Work out the finished part from the listing and answer in its coordinate system (mm). A direction names the side the tool comes from. Coordinates: 2 decimals unless noted, no trailing zeros. Order: outer loops, then holes, each group sorted by start corner. A loop starts at its lowest first (then second) coordinate and runs counter-clockwise, first axis right, second up. Notation, with made-up numbers: M 68.5,77.5 L 119.5,77.5 A12 ccw 119.5,83.5 Z; hole C 5,-29 d3. An arc over 180 degrees is marked long. Answer in a Markdown table with one row per item. Add a question column.
Item 1: Which of the six approach directions +Z, -Z, +X, -X, +Y, -Y give full straight-line access (tool end or side, diameter ignored) to faces 1 (the face through (9.5, 12, -23)), 2 (the face through (32, 15.25, -23)), 3 (the face through (0, 5.5, -23)), 4 (the face through (18, 15.75, -23))?
Item 2: Consider line 1 (X direction, y = 0.25, z = -9); line 2 (Z direction, x = 22, y = 18.25); line 3 (X direction, y = 16.65, z = -8). Determine where each line is inside the solid, lowest interval first. Write a range as from..to.
Item 3: The part is cut by section C-C (x = -4). Write down the section's boundary in (y, z), then the cut area to 3 significant figures.
Item 4: Flat-ended cylindrical pins translate along their axes: pin 1 Ø3.5 at (x, z) = (8, -19.5) entering from -Y; pin 2 Ø1.2 at (y, z) = (14.5, -13.5) entering from +X; pin 3 Ø1 at (x, z) = (13.5, -29) entering from -Y. Find the tip coordinate at first contact, or state that the pin passes through.
Item 5: The part is cut by section A-A (y = 0). Write down the section's boundary in (x, z).
Item 6: The mould has two halves that part along X. Classify faces 5 (the face through (12.5, 9, -23)), 6 (the face through (30, 13.75, -23)), 7 (the face through (9.5, -1, -23)): released by +X, released by -X, zero draft, split by the parting line, or undercut.
Item 7: The part is cut by section B-B (z = -8). State how many separate pieces and enclosed holes the cut face has, then the cut area to 3 significant figures.
Autodesk Inventor part; units mm, degrees
ref_plane "YZ Plane" through (0, 0, 0) normal (1, 0, 0) x (0, 1, 0)
ref_plane "XZ Plane" through (0, 0, 0) normal (0, 1, 0) x (-1, 0, 0)
ref_plane "XY Plane" through (0, 0, 0) normal (0, 0, 1) x (1, 0, 0)
sketch "Boceto1" plane through (0, 0, 0) normal (0, 0, 1) x (1, 0, 0)
  arc A0 (4.8153, 5.75) -> (4.8153, -5.75) centre (0, 0) ccw
  line L0 (0, 12.1119) -> (0, -11.4197) construction
  line L1 (-11.1817, 0) -> (12.1806, 0) construction
  line L2 (4.9434, 0.75) -> (5.5, 0.75)
  line L3 (4.9434, -0.75) -> (5.5, -0.75)
  line L4 (5.5, -0.75) -> (5.5, 0.75)
  line L5 (-0.75, 4.9434) -> (-0.75, 5.5)
  line L6 (0.75, 5.5) -> (-0.75, 5.5)
  line L7 (0.75, 4.9434) -> (0.75, 5.5)
  line L8 (-4.9434, -0.75) -> (-5.5, -0.75)
  line L9 (-5.5, 0.75) -> (-5.5, -0.75)
  line L10 (-4.9434, 0.75) -> (-5.5, 0.75)
  line L11 (0.75, -4.9434) -> (0.75, -5.5)
  line L12 (-0.75, -5.5) -> (0.75, -5.5)
  line L13 (-0.75, -4.9434) -> (-0.75, -5.5)
  arc A1 (-0.75, 4.9434) -> (-4.9434, 0.75) centre (0, 0) ccw
  arc A2 (-4.9434, -0.75) -> (-0.75, -4.9434) centre (0, 0) ccw
  arc A3 (0.75, -4.9434) -> (4.9434, -0.75) centre (0, 0) ccw
  arc A4 (4.9434, 0.75) -> (0.75, 4.9434) centre (0, 0) ccw
  circle A5 centre (0, 0) radius 5 construction
  line L14 (-11.772, 7.5) -> (14.517, 7.5) construction
  line L15 (-11.772, -7.5) -> (14.517, -7.5) construction
  line L16 (4.8153, 5.75) -> (7.5, 5.75)
  line L17 (9.5, 7.75) -> (9.5, 17.25)
  line L18 (12, 19.75) -> (27.0665, 19.75)
  line L19 (31.5, 15.25) -> (31.5, 15.25)
  line L20 (31, 15.75) -> (29.5, 15.75)
  line L21 (29, 15.25) -> (29, 13.75)
  line L22 (29, 13.75) -> (31, 13.75)
  line L23 (31.5, 13.25) -> (31.5, 12.25)
  line L24 (31, 11.75) -> (29.4417, 11.75)
  line L25 (27, 14.1917) -> (27, 14.25)
  line L26 (25.5, 15.75) -> (15, 15.75)
  line L27 (15, 15.75) -> (15, 15.25)
  line L28 (15, 15.25) -> (13, 15.25)
  line L29 (13, 15.25) -> (13, 15.75)
  line L30 (13, 15.75) -> (12.5, 15.75)
  line L31 (12.5, 15.75) -> (12.5, 2.4675)
  line L32 (12.2113, 2.0143) -> (9.5, 0.75)
  line L33 (9.5, 0.75) -> (9.5, -2.75)
  line L34 (9.5, -2.75) -> (12, -2.75)
  line L35 (12.5, -3.25) -> (12.5, -5.25)
  line L36 (12, -5.75) -> (4.8153, -5.75)
  line L37 (33.5, 15.25) -> (33.5, 16.75)
  line L38 (31.5, 15.25) -> (33.5, 15.25)
  arc A6 (31, 11.75) -> (31.5, 12.25) centre (31, 12.25) ccw
  arc A7 (31.5, 13.25) -> (31, 13.75) centre (31, 13.25) ccw
  arc A8 (31.5, 15.25) -> (31, 15.75) centre (31, 15.25) ccw
  arc A9 (29.5, 15.75) -> (29, 15.25) centre (29.5, 15.25) ccw
  arc A10 (27, 14.25) -> (25.5, 15.75) centre (25.5, 14.25) ccw
  arc A11 (27, 14.1917) -> (29.4417, 11.75) centre (29.4417, 14.1917) ccw
  arc A12 (12, 19.75) -> (9.5, 17.25) centre (12, 17.25) ccw
  arc A13 (12.2113, 2.0143) -> (12.5, 2.4675) centre (12, 2.4675) ccw
  arc A14 (12.5, -3.25) -> (12, -2.75) centre (12, -3.25) ccw
  arc A15 (12, -5.75) -> (12.5, -5.25) centre (12, -5.25) ccw
  arc A16 (7.5, 5.75) -> (9.5, 7.75) centre (7.5, 7.75) ccw
  line L39 (33.5, 16.75) -> (27.0665, 19.75)
  point P0 (31.5, 13.75)
  point P1 (31.5, 11.75)
  point P2 (27, 11.75)
  point P3 (27, 15.75)
  point P4 (12.5, -2.75)
  point P5 (12.5, -5.75)
  point P6 (-7.5, 0)
  point P7 (5.5, 0)
  dimension "d0" = 15
  dimension "d4" = 0.75
  dimension "d6" = 1.5
  dimension "d11" = 360
  dimension "d13" = 10
  dimension "d14" = 0.5
  dimension "d15" = 5
  dimension "d16" = 1.75
  dimension "d17" = 1.75
  dimension "d18" = 11.5
  dimension "d20" = 3
  dimension "d21" = 3
  dimension "d22" = 3
  dimension "d23" = 4
  dimension "d24" = 115
  dimension "d26" = 19
  dimension "d27" = 14
  dimension "d28" = 0.5
  dimension "d30" = 0.5
  dimension "d31" = 8
  dimension "d33" = 0.5
  dimension "d36" = 2
  dimension "d41" = 65
  dimension "d43" = 0.5
  dimension "d44" = 0.5
  dimension "d45" = 1.5
  dimension "d47" = 2.5
  dimension "d48" = 0.5
  dimension "d49" = 2
  dimension "d88" = 20
  dimension "d89" = 4
  dimension "d92" = 27.25
  dimension "d93" = 2
  dimension "d94" = 2
  dimension "d95" = 14.5
  dimension "d96" = 2.4417
  dimension "d98" = 155
  dimension "d99" = 2
  dimension "d101" = 1.5
  dimension "d102" = 2.5
  dimension "d103" = 24
extrude "Extrusión1" add sketch "Boceto1" against normal blind 46
sketch "Boceto2" plane through (12, 19.75, 0) normal (0, 1, 0) x (1, 0, 0)
  line L0 (9.4815, 49.0857) -> (9.4815, -3.1706) construction
  line L1 (20.8474, 23) -> (-1.8844, 23) construction
  line L2 (0, 0) -> (0, 46) construction
  line L3 (15.0665, 0) -> (0, 0) construction
  line L4 (0, 46) -> (15.0665, 46) construction
  circle A0 centre (9.4815, 23) radius 2.5
  circle A1 centre (9.4815, 23) radius 4.5
  circle A2 centre (9.4815, 8) radius 2.5
  circle A3 centre (9.4815, 8) radius 4.5
  circle A4 centre (9.4815, 38) radius 2.5
  circle A5 centre (9.4815, 38) radius 4.5
  line L5 (15.0665, 0) -> (15.0665, 46)
  point P0 (-12, 0)
  dimension "d67" = 23
  dimension "d68" = 23
  dimension "d69" = 5
  dimension "d70" = 9
  dimension "d72" = 2
  dimension "d75" = 15
  dimension "d104" = 5.585
hole "Agujero1" at (21.4815, 19.75, -38) at (21.4815, 19.75, -23) at (21.4815, 19.75, -8) direction (0, -1, 0) diameter 5 end through all countersink diameter 9 countersink angle 90
properties part number "HIN-61 BISAGRA" material "Aluminio"
Reply:
| question | item | result |
|---|---|---|
| 1 | face 1 | +Z, -Z, -X, +Y |
| 1 | face 2 | +Z, -Z, +X, -Y |
| 1 | face 3 | +Z, -Z |
| 1 | face 4 | +Z, -Z, -Y |
| 2 | line 1 | x = -7.5..-5.5, 5.5..9.5 |
| 2 | line 2 | z = -46..-40.95, -35.05..-25.95, -20.05..-10.95, -5.05..0 |
| 2 | line 3 | x = 9.5..18.98, 23.98..33.5 |
| 3 | outline | M -6.34,-46 L -3,-46 L -3,0 L -6.34,0 Z; M 3,-46 L 6.34,-46 L 6.34,0 L 3,0 Z |
| 3 | area | 308 mm2 |
| 4 | pin 1 | stops at y = -5.75 |
| 4 | pin 2 | stops at x = 29 |
| 4 | pin 3 | stops at y = 15.25 |
| 5 | outline | M -7.5,-46 L -5.5,-46 L -5.5,0 L -7.5,0 Z; M 5.5,-46 L 9.5,-46 L 9.5,0 L 5.5,0 Z |
| 6 | face 5 | undercut |
| 6 | face 6 | zero draft |
| 6 | face 7 | released by +X |
| 7 | separate pieces | 2 |
| 7 | enclosed holes | 1 |
| 7 | area | 255 mm2 |
